Job drawing, mm, ordinate dimensions from the low corner. One solid piece. A direction names the side the tool comes from. Coordinates: 2 decimals unless noted, no trailing zeros. Order: outer loops, then holes, each group sorted by start corner. A loop starts at its lowest first (then second) coordinate and runs counter-clockwise, first axis right, second up. Notation, with made-up numbers: M 82.25,-23 L 135.25,-23 A10 cw 135.25,-12 Z; hole C 3.5,-16 d10. An arc over 180 degrees is marked long. Write item = value, one per line.
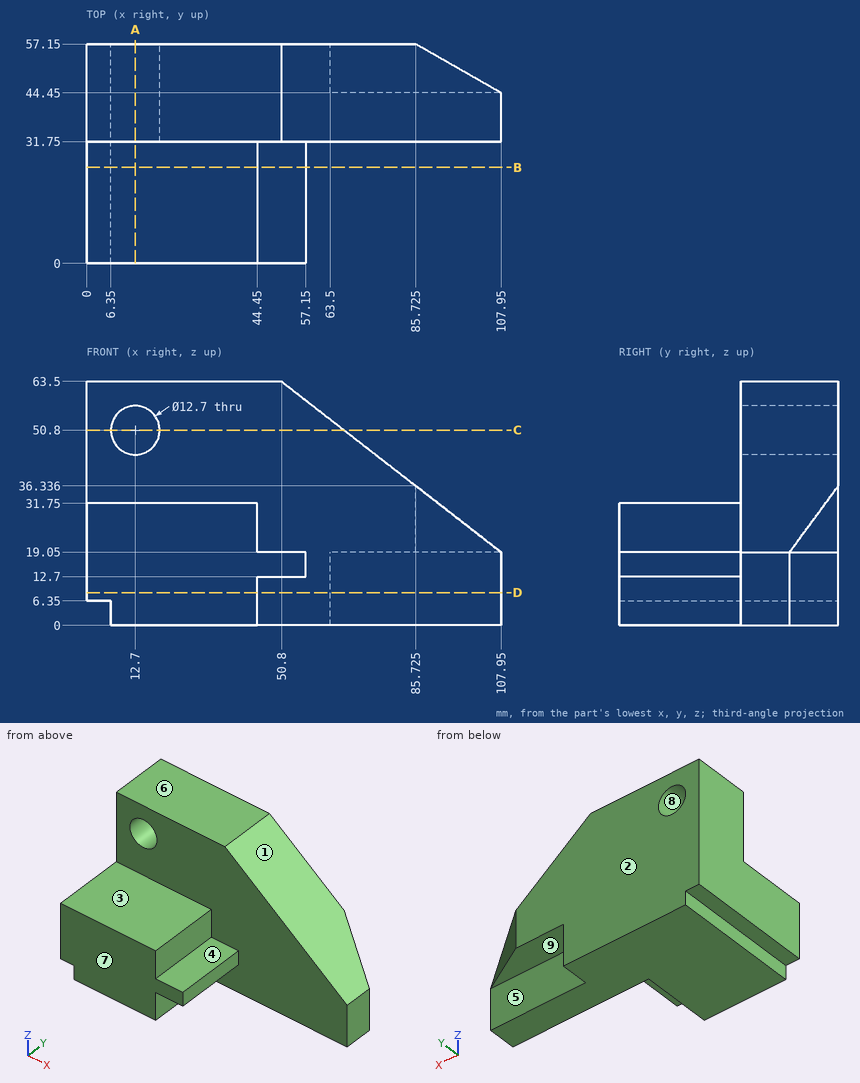
(1) Tool access for the marked faces 1, 2, 3, 4 and 5: list every direction of +Z, -Z, +X, -X, +Y, -Y with a clear straight run to the whole face (end or side of a thin tool).
Evaluation:
face_1 = +Z, +X, +Y, -Y
face_2 = +Z, -Z, +X, -X, +Y
face_3 = +Z, +X, -X, -Y
face_4 = +Z, +X, -Y
face_5 = -Z, +X, +Y
(2) Pin check, flat tips, straight feed: pin 1 Ø6.5 at (x, y) = (49.5, 12.5) entering from -Z; pin 2 Ø10 at (y, z) = (9, 4) entering from +X; pin 3 Ø3 at (x, y) = (72, 32) entering from +Z. Stop position of each tip, or through.
Evaluation:
pin_1 = 12.7
pin_2 = 44.45
pin_3 = 48.18
(3) Slice it at D-D, the plane z = 8.5. Write the cut outline in (x, y), then the cut area to 3 significant figures.
Evaluation:
outline = M 0,0 L 44.45,0 L 44.45,31.75 L 107.95,31.75 L 107.95,44.45 L 63.5,44.45 L 63.5,57.15 L 0,57.15 Z
area = 3,590 mm²
(4) Slice it at A-A, the plane x = 12.7. Write the cut outline in (y, z).
Evaluation:
outline = M 0,0 L 57.15,0 L 57.15,44.45 L 31.75,44.45 L 31.75,31.75 L 0,31.75 Z; M 31.75,57.15 L 57.15,57.15 L 57.15,63.5 L 31.75,63.5 Z
(5) Slice it at B-B, the plane y = 25. Write the cut outline in (x, z), then the cut area to 3 significant figures.
Evaluation:
outline = M 0,6.35 L 6.35,6.35 L 6.35,0 L 44.45,0 L 44.45,12.7 L 57.15,12.7 L 57.15,19.05 L 44.45,19.05 L 44.45,31.75 L 0,31.75 Z
area = 1,450 mm²
(6) Wall check: line 1 (Z direction, x = 12.7, y = 47.75); line 2 (Y direction, x = 77.5, z = 7.5); line 3 (Y direction, x = 52, z = 34). Give the ranges that are in metal, low to high. Write a range as from..to.
Evaluation:
line_1 = 0..44.45, 57.15..63.5
line_2 = 31.75..44.45
line_3 = 31.75..57.15
(7) Pull direction Z, two halves, no side cores. Call the marked faces 6, 7, 8 and 9: +Z half, -Z half, draft (parallel to the pull), parting line (faces both ways), or undercut.
Evaluation:
face_6 = +Z half
face_7 = draft
face_8 = undercut
face_9 = -Z half
(8) Slice it at C-C, the plane z = 50.8. Write the cut outline in (x, y).
Evaluation:
outline = M 0,31.75 L 6.35,31.75 L 6.35,57.15 L 0,57.15 Z; M 19.05,31.75 L 67.13,31.75 L 67.13,57.15 L 19.05,57.15 Z
